Geometry check sheet. Reference: the model listing, model coordinates, mm. Face numbers are marked on the shaded views. A direction names the side the tool comes from. Give positions to 0.01 mm unless a question says otherwise; leave off trailing zeros. Order: outer loops, then holes, each group sorted by start corner. A loop starts at its lowest first (then second) coordinate and runs counter-clockwise, first axis right, second up. Notation, with made-up numbers: M 63.25,-37.75 L 104.25,-37.75 A22 ccw 104.25,-24.75 Z; hole C -19,-16.75 d2. An arc over 180 degrees is marked long. Answer as CSV lines item,"result".
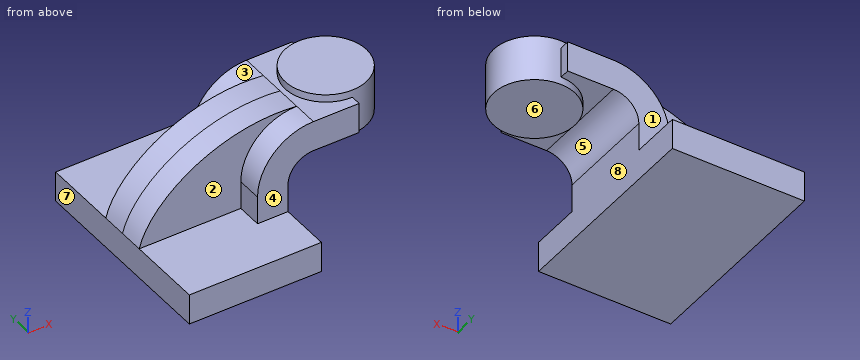
from build123d import *

# Parameters (mm, degrees)
F1_DEPTH = 63.5
F0_W     = 25.4
F0_H     = 19.05
F2_DEPTH = 31.75
F4_DEPTH = 15.875


with BuildPart() as f1:
    # F0 (on Front) → F1 (new body, symmetric)
    with BuildSketch(Plane.XZ):
        Polygon((22.225, 9.525), (-41.275, 9.525), (-41.275, -9.525), (41.275, -9.525), (41.275, 9.525), align=None)
    extrude(amount=F1_DEPTH, both=True)

    # F0 (on Front) → F2 (join, symmetric)
    with BuildSketch(Plane.XZ):
        with BuildLine():
            Line((22.225, 27.0002), (22.225, 9.525))
            Line((22.225, 9.525), (41.275, 9.525))
            Line((41.275, 9.525), (41.275, 27.0002))
            ThreePointArc((41.275, 27.0002), (45.9246798487, 38.2255201513), (57.15, 42.8752))
            Line((57.15, 42.8752), (60.325, 42.8752))
            Line((60.325, 42.8752), (60.325, 61.9252))
            Line((60.325, 61.9252), (57.15, 61.9252))
            ThreePointArc((57.15, 61.9252), (32.4542956671, 51.6959043329), (22.225, 27.0002))
        make_face()
        with Locations((73.025, 52.4002)):
            Rectangle(F0_W, F0_H)
    extrude(amount=F2_DEPTH, both=True)

    # F0 (on Front) → F3 (revolve)
    with BuildSketch(Plane.XZ):
        Polygon((85.725, 66.675), (85.725, 61.9252), (85.725, 42.8752), (85.725, 38.1), (111.125, 38.1), (111.125, 66.675), align=None)
    revolve(axis=Axis((85.725, 0, 52.3875), (0, 0, 1)))

    # F0 (on Front) → F4 (join, symmetric)
    with BuildSketch(Plane.XZ):
        with BuildLine():
            add(Edge.make_bspline(
                [(-41.275, 9.525), (-34.2721380293, 37.1860302985), (7.8561343253, 67.5534531474), (57.15, 61.9252)],
                knots=[0, 0, 0, 0, 111.5045361635, 111.5045361635, 111.5045361635, 111.5045361635], degree=3))
            Line((-41.275, 9.525), (22.225, 9.525))
            Line((22.225, 9.525), (22.225, 27.0002))
            ThreePointArc((22.225, 27.0002), (32.4542956671, 51.6959043329), (57.15, 61.9252))
        make_face()
    extrude(amount=F4_DEPTH, both=True)


solid = f1.part
(1) Section check A-A on y = 29.5. Enter the section's corners in (x, z) (3 decimals), then the cut area to 3 significant figures.
The answers:
outline,"M -41.275,-9.525 L 41.275,-9.525 L 41.275,27 A15.875 cw 57.15,42.875 L 85.725,42.875 L 85.725,61.925 L 57.15,61.925 A34.925 ccw 22.225,27 L 22.225,9.525 L -41.275,9.525 Z"
area,"3,210 mm2"
(2) Draft check along X on the marked faces 5, 6, 7 and 8. Enter one of: +X half, -X half, draft (parallel to the pull), parting line (faces both ways), or undercut.
The answers:
face 5,"undercut"
face 6,"draft"
face 7,"-X half"
face 8,"+X half"
(3) Section check C-C on y = -54.5. Enter the section's corners in (x, z) (3 decimals).
The answers:
outline,"M -41.275,-9.525 L 41.275,-9.525 L 41.275,9.525 L -41.275,9.525 Z"
(4) Gauge pin test, flat ends, axial feed: P1, Ø15.5, axis at x = 48, z = 45, coming from the -Y side; P2, Ø7, axis at y = 29, z = 52.5, coming from the +X side (3 decimals); P3, Ø15.5, axis at x = 63.5, z = 40, coming from the +Y side; P4, Ø17.5, axis at y = 26.5, z = 14.5, coming from the -X side (3 decimals). Record the tip position at first contact, or that the pin passes through.
The answers:
P1,"stops at y = -31.75"
P2,"stops at x = 85.725"
P3,"stops at y = 31.75"
P4,"stops at x = -41.275"
(5) Tool access check on the marked faces 1, 2, 3 and 4. Record the directions out of +Z, -Z, +X, -X, +Y, -Y that give a thin tool (end or side, any length) a straight path to the whole face; none if there is none.
The answers:
face 1,"+Z, +X, -X, +Y"
face 2,"+Z, -X, -Y"
face 3,"+Z, -X, +Y"
face 4,"+Z, +X, -X, -Y"
(6) Section check B-B on z = 3.5. Enter the section's corners in (x, y) (3 decimals).
The answers:
outline,"M -41.275,-63.5 L 41.275,-63.5 L 41.275,63.5 L -41.275,63.5 Z"
(7) Material ranges on line 1 (Y direction, x = -6.5, z = 37.5) (3 decimals); line 2 (Z direction, x = -31, y = -35) (3 decimals); line 3 (Z direction, x = 59, y = 10), recorded low to high.
The answers:
line 1,"y = -15.875 to 15.875"
line 2,"z = -9.525 to 9.525"
line 3,"z = 42.88 to 61.93"
